Work out the finished part from the listing and answer in its coordinate system (mm). Face numbers are marked on the shaded views. A direction names the side the tool comes from. Give positions to 0.01 mm unless a question says otherwise; leave off trailing zeros. Loops run counter-clockwise (first coordinate to the right, second up) from the corner with the lowest first, then second, coordinate; pieces in that order, holes last. Notation, with made-up numbers: (39.25, 44) -> (69.25, 44) arc R21 cw to (69.25, 63) -> close; hole circle Ø10 at (70.5, 1). An arc over 180 degrees is marked (long way). Answer as CSV lines item,"result". Start each with the question number.
1. Flat-ended cylindrical pins translate along their axes: pin 1 Ø5 at (y, z) = (-5.29, -7.28) entering from -X; pin 2 Ø7 at (y, z) = (0, 9) entering from +X; pin 3 Ø4 at (x, z) = (1.5, -11.5) entering from +Y; pin 4 Ø3 at (x, z) = (6, 13) entering from -Y. Find the tip coordinate at first contact, or state that the pin passes through.
2. A tool of negligible diameter and unlimited length cuts with its end or side. For the marked faces 1 and 2, from which of +Z, -Z, +X, -X, +Y, -Y can it reach the whole face along a straight path? Write none if from no direction.
3. Find section A-A, the plane y = 0. Give the vertices of the cut face in (x, z).
4. Find section C-C, the plane x = 0.75. Give the vertices of the cut face in (y, z), and give its area (3 significant figures).
5. Find section B-B, the plane x = 4.25. Give the vertices of the cut face in (y, z).
6. Find section D-D, the plane z = 0.5. Count the separate pieces of the cut face and the enclosed holes in it, and give its area (3 significant figures).
7. Determine the mould class of the marked faces 3, 4 and 5 for opening direction Y: +Y half, -Y half, draft (parallel to the pull), parting line (faces both ways), or undercut.
8. Find the intervals of material crossed by line 1 along Z through (x, y) = (0.95, 0); line 2 along Z through (x, y) = (7.5, -1); line 3 along Z through (x, y) = (1.75, 1), in increasing order.
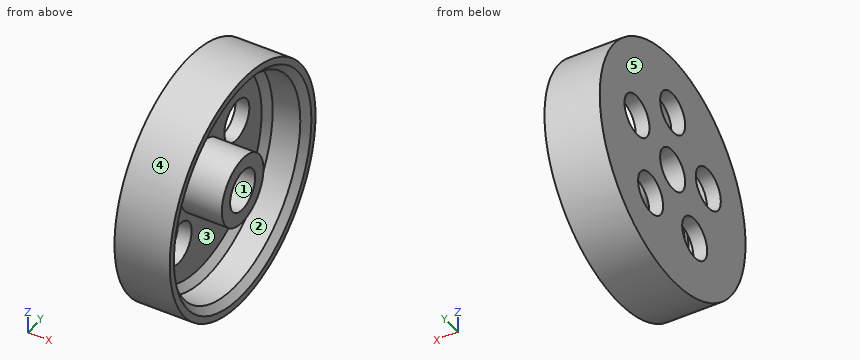
from build123d import *

# Parameters (mm, degrees)
F0_W            = 8
F0_H            = 17.5
F3_D            = 6
F4_T            = -2
F5_SIZE         = 1
F7_D            = 6
F7_COPIES_COUNT = 5


# Not quite as in the source:
# - a pattern or mirror of a feature is missing from the dataset's text; its kind, count and spacing are read off the source's solid


with BuildPart() as f1:
    # F0 (on Top) → F1 (revolve)
    with BuildSketch(Plane.XY):
        with Locations((4, 8.75)):
            Rectangle(F0_W, F0_H)
    revolve(axis=Axis((4, 0, 0), (1, 0, 0)))

    # F3 (through all)
    with Locations(Plane(origin=(0, 0, 0), x_dir=(0, 1, 0), z_dir=(-1, 0, 0))):
        with Locations((0, 0)):
            Hole(F3_D / 2)

    # F4
    f4_openings = [f1.faces().sort_by_distance(p)[0] for p in [
        (8, -17.005025, 0),
    ]]
    offset(amount=F4_T, openings=f4_openings)

    # F5
    f5_edges = [f1.edges().sort_by_distance(p)[0] for p in [
        (8, -15.5, 0),
        (5, 15.5, 0),
        (2, -15.5, 0),
    ]]
    chamfer(f5_edges, length=F5_SIZE)

    # F7 (through all)
    with Locations(Plane(origin=(0, 0, 0), x_dir=(0, 1, 0), z_dir=(-1, 0, 0))):
        with Locations((0, -9)):
            f7 = Hole(F7_D / 2)

    # F7_copies: F7 ×5 about axis
    f7_copies_axis = Axis((0, 0, 0), (1, 0, 0))
    for i in range(1, F7_COPIES_COUNT):
        add(f7.rotate(f7_copies_axis, i * 360 / F7_COPIES_COUNT), mode=Mode.SUBTRACT)


solid = f1.part
Resolved:
1,pin 1,"passes through"
1,pin 2,"stops at x = 2"
1,pin 3,"stops at y = 14.7"
1,pin 4,"stops at y = -13.19"
2,face 1,"+X, -X"
2,face 2,"+X"
3,outline,"(0, -17.5) -> (8, -17.5) -> (8, -16.5) -> (7, -15.5) -> (3, -15.5) -> (2, -14.5) -> (2, -5) -> (8, -5) -> (8, -3) -> (0, -3) -> close; (0, 3) -> (8, 3) -> (8, 5) -> (2, 5) -> (2, 6) -> (0, 6) -> close; (0, 12) -> (2, 12) -> (2, 14.5) -> (3, 15.5) -> (7, 15.5) -> (8, 16.5) -> (8, 17.5) -> (0, 17.5) -> close"
4,outline,"circle Ø35 at (0, 0); hole circle Ø6 at (-8.56, 2.78); hole circle Ø6 at (-5.29, -7.28); hole circle Ø6 at (0, 0); hole circle Ø6 at (0, 9); hole circle Ø6 at (5.29, -7.28); hole circle Ø6 at (8.56, 2.78)"
4,area,"792 mm^2"
5,outline,"circle Ø35 at (0, 0); circle Ø10 at (0, 0); hole circle Ø31 at (0, 0); hole circle Ø6 at (0, 0)"
6,separate pieces,"4"
6,enclosed holes,"0"
6,area,"90.8 mm^2"
7,face 3,"undercut"
7,face 4,"parting line"
7,face 5,"draft"
8,line 1,"z = -17.5 to -3, 3 to 6, 12 to 17.5"
8,line 2,"z = -17.47 to -15.97, -4.9 to -2.83, 2.83 to 4.9, 15.97 to 17.47"
8,line 3,"z = -17.47 to -2.83, 2.83 to 6.17, 11.83 to 17.47"
